Check sheet for the modelled part. Datum: model origin and axes. Units: mm. Coordinates: 2 decimals unless noted, no trailing zeros. Loops run counter-clockwise (first coordinate to the right, second up) from the corner with the lowest first, then second, coordinate; pieces in that order, holes last. Notation, with made-up numbers: (79.5, 9) -> (95.5, 9) arc R27 cw to (95.5, 34) -> close; hole circle Ø1 at (-0.5, -20.75). An arc over 180 degrees is marked (long way). Use CSV: the item, a comma, the result in double quotes.
```python
from build123d import *

# Parameters (mm, degrees)
CYLINDER_R           = 1.5
CYLINDER_DEPTH       = 10
CYLINDER_PITCH_ANGLE = 90


with BuildPart() as screwcutout:
    # Cylinder → Cylinder (new body)
    with BuildSketch(Plane.XY):
        Circle(CYLINDER_R)
    extrude(amount=CYLINDER_DEPTH)


with BuildPart() as screwcutout_1:
    # Cylinder pitch: moved
    add(screwcutout.part.rotate(Axis((0, 0, 0), (0, 1, 0)), CYLINDER_PITCH_ANGLE))


with BuildPart() as screwcutout_2:
    # Cylinder placement: moved
    add(screwcutout_1.part)


with BuildPart() as innerrace001:
    # Sketch002 → Revolution002 (revolve)
    with BuildSketch(Plane.XZ):
        Polygon((0, 3.346519), (2.853732, 6.200251), (3.853732, 6.200251), (3.853732, 0), (0, 0), align=None)
    revolve(axis=Axis((0, 0, 0), (1, 0, 0)))

    # Cut002: cut ScrewCutout
    add(screwcutout_2.part, mode=Mode.SUBTRACT)


solid = innerrace001.part
```
1) Go/stop test with flat-tipped pins: pin 1 Ø1.5 at (x, y) = (1.5, 3.5) entering from +Z; pin 2 Ø2 at (x, z) = (1, -1.5) entering from +Y. Record where each tip stops, or that it passes through.
Answer below:
pin 1,"stops at z = 4.52"
pin 2,"stops at y = 5.17"
2) Cross-section at D-D on x = 1.8. Record the boundary of the cut face in (y, z).
Answer below:
outline,"circle Ø10.29 at (0, 0); hole circle Ø3 at (0, 0)"
3) Cross-section at C-C on x = 3.2. Record the boundary of the cut face in (y, z).
Answer below:
outline,"circle Ø12.4 at (0, 0); hole circle Ø3 at (0, 0)"
4) Draft check along Z on faces 1 (the flat face through (0, -2, 0)), 2 (the cylindrical face through (3.361, 6.053, -1.344)), 3 (the cylindrical face through (1.9, -0.9, 1.2)). Enter one of: released by +Z, released by -Z, zero draft, split by the parting line, or undercut.
Answer below:
face 1,"zero draft"
face 2,"split by the parting line"
face 3,"undercut"
5) Thickness scan on line 1 along Z through (x, y) = (2.95, 0); line 2 along Y through (x, z) = (2.4, -0.5); line 3 along Y through (x, z) = (2.8, 0). Record the ranges inside material, lowest first. Write a range as from..to.
Answer below:
line 1,"z = -6.2..-1.5, 1.5..6.2"
line 2,"y = -5.72..-1.41, 1.41..5.72"
line 3,"y = -6.15..-1.5, 1.5..6.15"
6) Cross-section at A-A on y = 0. Record the boundary of the cut face in (x, z), and give its area (3 significant figures).
Answer below:
outline,"(0, -3.35) -> (2.85, -6.2) -> (3.85, -6.2) -> (3.85, -1.5) -> (0, -1.5) -> close; (0, 1.5) -> (3.85, 1.5) -> (3.85, 6.2) -> (2.85, 6.2) -> (0, 3.35) -> close"
area,"28.1 mm²"
